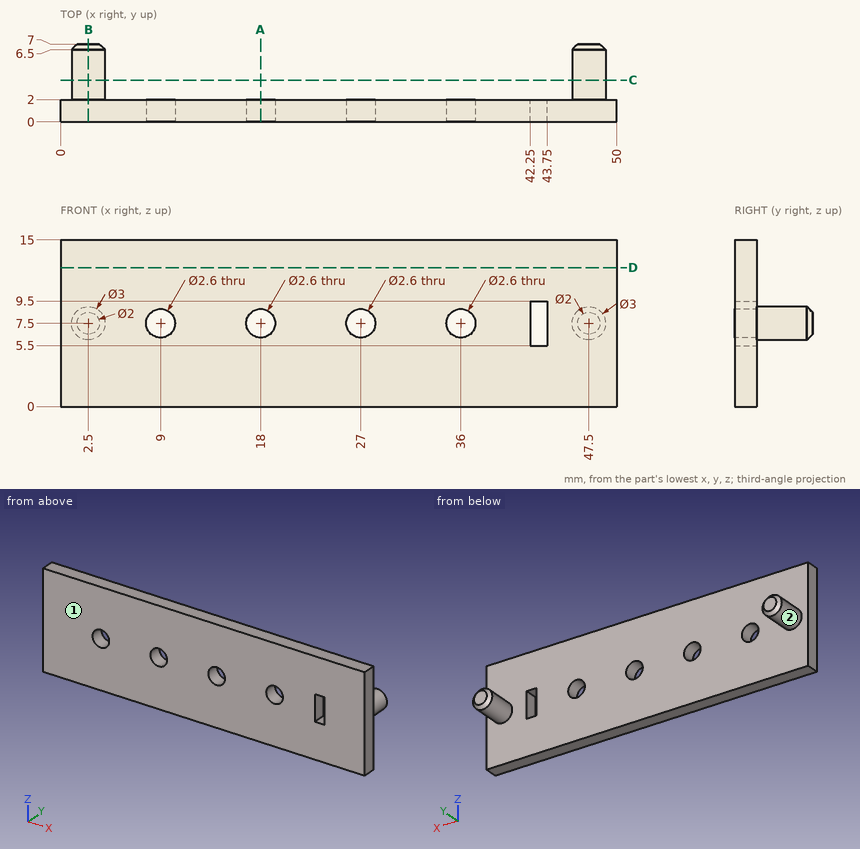
Check sheet for the drawn part. Datum: minimum x, y, z corner. Units: mm. A direction names the side the tool comes from. Round coordinates to 2 decimals unless told otherwise and drop trailing zeros. Order: outer loops, then holes, each group sorted by start corner. A loop starts at its lowest first (then second) coordinate and runs counter-clockwise, first axis right, second up.
(1) Scan lines: probe 1 along X at (y, z) = (1.25, 7.5); probe 2 along Y at (x, z) = (25.5, 11.25); probe 3 along X at (y, z) = (3.5, 7.25). Record each from-to range of solid material in increasing order.
(2) Cross-section at D-D, the plane z = 12.5. Enter the section's corners in (x, y), and give its area (3 significant figures).
(3) Cross-section at A-A, the plane x = 18. Enter the section's corners in (y, z), and give its area (3 significant figures).
(4) Go/stop test with a flat-tipped pin: P1, Ø1, axis at x = 8.5, z = 5, coming from the +Y side. Record where the tip stops, or that it passes through.
(5) Access from +Z, -Z, +X, -X, +Y, -Y to the whole of each face (thin tool, end or side, straight path). Record for the marked faces 1 and 2.
(6) Cross-section at C-C, the plane y = 3.75. Enter the section's corners in (x, z), and give its area (3 significant figures).
(7) Cross-section at B-B, the plane x = 2.5. Enter the section's corners in (y, z).
Check sheet entries:
1. probe 1: x = 0 to 7.7, 10.3 to 16.7, 19.3 to 25.7, 28.3 to 34.7, 37.3 to 42.25, 43.75 to 50
1. probe 2: y = 0 to 2
1. probe 3: x = 1.02 to 3.98, 46.02 to 48.98
2. outline: (0, 0) - (50, 0) - (50, 2) - (0, 2) - close
2. area: 100 mm2
3. outline: (0, 0) - (2, 0) - (2, 6.2) - (0, 6.2) - close; (0, 8.8) - (2, 8.8) - (2, 15) - (0, 15) - close
3. area: 24.8 mm2
4. P1: stops at y = 2
5. face 1: +Z, -Z, +X, -X, -Y
5. face 2: +Y
6. outline: circle Ø3 at (2.5, 7.5); circle Ø3 at (47.5, 7.5)
6. area: 14.1 mm2
7. outline: (0, 0) - (2, 0) - (2, 6) - (6.5, 6) - (7, 6.5) - (7, 8.5) - (6.5, 9) - (2, 9) - (2, 15) - (0, 15) - close
